from build123d import *

# Parameters (mm, degrees)
F1_DEPTH = 275
F3_DEPTH = 3.7


with BuildPart() as f1:
    # F0 (on Front) → F1 (new body)
    with BuildSketch(Plane.XZ):
        Polygon((0, 41), (0, 0), (41, 0), (41, 41), (31.4, 41), (31.4, 34), (34.8, 34), (34.8, 37.5), (37.3, 37.5), (37.3, 3.7), (3.7, 3.7), (3.7, 37.5), (6.2, 37.5), (6.2, 34), (9.6, 34), (9.6, 41), align=None)
    extrude(amount=F1_DEPTH)

    # F2 (on face) → F3 (cut, through all)
    with BuildSketch(Plane(origin=(0, 0, 0), x_dir=(1, 0, 0), z_dir=(0, 0, -1))):
        with BuildLine():
            Line((15.5, 255), (15.5, 20))
            ThreePointArc((15.5, 20), (20.5, 15), (25.5, 20))
            Line((25.5, 20), (25.5, 255))
            ThreePointArc((25.5, 255), (20.5, 260), (15.5, 255))
        make_face()
    extrude(amount=-F3_DEPTH, mode=Mode.SUBTRACT)


solid = f1.part
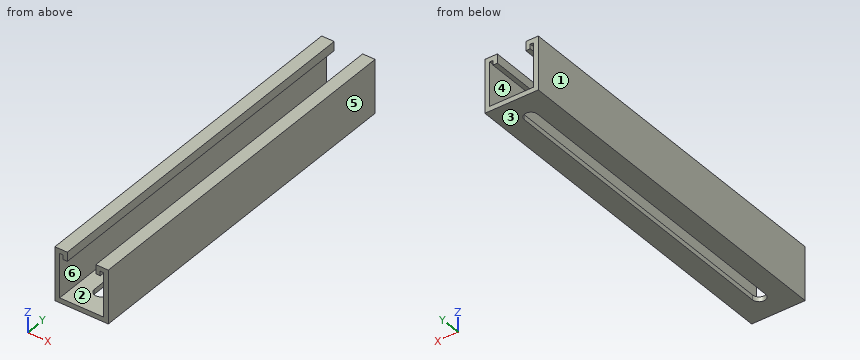
For this review, take the finished solid that the model builds, in its own axes (mm). Face numbers are marked on the shaded views. A direction names the side the tool comes from. Round coordinates to 2 decimals unless told otherwise and drop trailing zeros. Loops run counter-clockwise (first coordinate to the right, second up) from the corner with the lowest first, then second, coordinate; pieces in that order, holes last. Notation, with made-up numbers: (30.5, -17) - (87.5, -17) arc R20 cw to (87.5, -12) - close; hole circle Ø9 at (-35, -17). An arc over 180 degrees is marked (long way). One line per item, written item: value. Start each with the question number.
Item 1: Take a section at C-C (x = 20.5). Give the boundary of the cut face in (y, z), plus the area to 3 significant figures.
Item 2: For the marked faces 5 and 6, list the 3-axis set-ups (+Z, -Z, +X, -X, +Y, -Y) from which the entire face can be reached by the end or side of a thin tool; tool diameter is ignored.
Item 3: Clearance check with a flat-ended pin moving along its axis: pin 1 Ø10 at (x, y) = (23.5, -234) entering from +Z. State where the tip first meets the part, or that it passes through.
Item 4: For L1, parallel to X at y = -227, z = 31; L2, parallel to Z at x = 9, y = -49.5; L3, parallel to X at y = -164.5, z = 39, list the stretches that pass through material, from the lowest coordinate up.
Item 5: The part is to be moulded in two halves that separate along Z. For the marked faces 1, 2, 3 and 4, say which applies: +Z half, -Z half, draft (parallel to the pull), parting line (faces both ways), or undercut.
Item 6: Take a section at A-A (y = -152.5). Give the boundary of the cut face in (x, z), plus the area to 3 significant figures.
Item 7: Take a section at B-B (z = 18.5). Give the boundary of the cut face in (x, y), plus the area to 4 significant figures.
Answer below:
1. outline: (-275, 0) - (-260, 0) - (-260, 3.7) - (-275, 3.7) - close; (-15, 0) - (0, 0) - (0, 3.7) - (-15, 3.7) - close
1. area: 111 mm2
2. face 5: +Z, -Z, +X, +Y, -Y
2. face 6: +Y, -Y
3. pin 1: stops at z = 3.7
4. L1: x = 0 to 3.7, 37.3 to 41
4. L2: z = 0 to 3.7, 34 to 41
4. L3: x = 0 to 9.6, 31.4 to 41
5. face 1: draft
5. face 2: undercut
5. face 3: -Z half
5. face 4: undercut
6. outline: (0, 0) - (15.5, 0) - (15.5, 3.7) - (3.7, 3.7) - (3.7, 37.5) - (6.2, 37.5) - (6.2, 34) - (9.6, 34) - (9.6, 41) - (0, 41) - close; (25.5, 0) - (41, 0) - (41, 41) - (31.4, 41) - (31.4, 34) - (34.8, 34) - (34.8, 37.5) - (37.3, 37.5) - (37.3, 3.7) - (25.5, 3.7) - close
6. area: 456 mm2
7. outline: (0, -275) - (3.7, -275) - (3.7, 0) - (0, 0) - close; (37.3, -275) - (41, -275) - (41, 0) - (37.3, 0) - close
7. area: 2,035 mm2
